Verification items for the finished model (mm, model axes). Coordinates: 2 decimals unless noted, no trailing zeros. Order: outer loops, then holes, each group sorted by start corner. A loop starts at its lowest first (then second) coordinate and runs counter-clockwise, first axis right, second up. Notation, with made-up numbers: M -17,5.25 L 6,5.25 A31 ccw 6,31.25 Z; hole C 72.5,-32 d8. An arc over 180 degrees is marked long. Use one line per item in the form item = value. Start each with the question number.
```python
from build123d import *

# Parameters (mm, degrees)
SKETCH_R  = 1.651
PAD_DEPTH = 2


with BuildPart() as part:
    # Sketch → Pad (new body)
    with BuildSketch(Plane.XY):
        with BuildLine():
            Line((-3.5, 45.4), (-3.5, -45.4))
            ThreePointArc((-3.5, -45.4), (-2.914214, -46.814214), (-1.5, -47.4))
            Line((-1.5, -47.4), (1.5, -47.4))
            Line((1.5, -47.4), (3.5, -47.4))
            Line((4.499988, -47.400006), (3.5, -47.4))
            ThreePointArc((4.499988, -47.400006), (5.914209, -46.814224), (6.5, -45.400006))
            Line((6.5, 45.4), (6.5, -45.400006))
            ThreePointArc((6.5, 45.4), (5.914214, 46.814214), (4.5, 47.4))
            Line((3.5, 47.4), (4.5, 47.4))
            Line((1.5, 47.4), (3.5, 47.4))
            Line((1.5, 47.4), (-1.5, 47.4))
            ThreePointArc((-1.5, 47.4), (-2.914214, 46.814214), (-3.5, 45.4))
        make_face()
        with Locations((0, 23.7)):
            Circle(SKETCH_R, mode=Mode.SUBTRACT)
        with Locations((0, -23.7)):
            Circle(SKETCH_R, mode=Mode.SUBTRACT)
    extrude(amount=PAD_DEPTH)


solid = part.part
```
1. Release check for a two-part mould opening along Y. For faces 1 (the flat face through (1, 1, 0)), 2 (the cylindrical face through (0.762, 22.235, 0.986)), 3 (the flat face through (2, 47.4, 1)) record: pulls with the +Y half, pulls with the -Y half, needs draft (parallel to the pull), parting line crosses it, or undercut.
2. Cross-section at A-A on y = 23.7. Enter the section's corners in (x, z), and give its area (3 significant figures).
3. Cross-section at C-C on z = 1.05. Enter the section's corners in (x, y).
4. Cross-section at B-B on x = 0. Enter the section's corners in (y, z).
5. Material ranges on line 1 along Y through (x, z) = (0, 1.1); line 2 along Y through (x, z) = (1.25, 0.9); line 3 along X through (y, z) = (-24.5, 1.85), recorded low to high.
Final values:
q1.face_1 = needs draft
q1.face_2 = undercut
q1.face_3 = pulls with the +Y half
q2.outline = M -3.5,0 L -1.65,0 L -1.65,2 L -3.5,2 Z; M 1.65,0 L 6.5,0 L 6.5,2 L 1.65,2 Z
q2.area = 13.4 mm2
q3.outline = M -3.5,-45.4 A2 ccw -1.5,-47.4 L 3.5,-47.4 L 4.5,-47.4 A2 ccw 6.5,-45.4 L 6.5,45.4 A2 ccw 4.5,47.4 L -1.5,47.4 A2 ccw -3.5,45.4 Z; hole C 0,-23.7 d3.3; hole C 0,23.7 d3.3
q4.outline = M -47.4,0 L -25.35,0 L -25.35,2 L -47.4,2 Z; M -22.05,0 L 22.05,0 L 22.05,2 L -22.05,2 Z; M 25.35,0 L 47.4,0 L 47.4,2 L 25.35,2 Z
q5.line_1 = -47.4 to -25.35, -22.05 to 22.05, 25.35 to 47.4
q5.line_2 = -47.4 to -24.78, -22.62 to 22.62, 24.78 to 47.4
q5.line_3 = -3.5 to -1.44, 1.44 to 6.5
